Source: CAD feature listing. Evaluate the final solid. Frame: model axes, mm. A direction names the side the tool comes from. Coordinates: 2 decimals unless noted, no trailing zeros. Loops run counter-clockwise (first coordinate to the right, second up) from the corner with the lowest first, then second, coordinate; pieces in that order, holes last. Notation, with made-up numbers: M 7,-22.5 L 59,-22.5 A34 ccw 59,14.5 Z; hole C -15,16 d3. An arc over 180 degrees is marked long. One line per question, with ' | ' between items. Start each with the question number.
1. Section query C-C, the plane z = -0.5. Output: boundary loops of the cut face in (x, y).
2. Section query D-D, the plane x = -33. Output: boundary loops of the cut face in (y, z), and give its area (3 significant figures).
3. Mould query, pull axis Y, two halves, no side actions, for faces 4 (the flat face through (1, 80, -25)), 5 (the flat face through (-55, 32, -14)), 6 (the flat face through (26, 58, -16.876)), 7 (the cylindrical face through (20.24, 51.35, -14.34)). Classes: pulls with the +Y half, pulls with the -Y half, needs draft (parallel to the pull), parting line crosses it, or undercut.
4. Pin query (flat end, axial travel): P1, Ø5, axis at x = -19.5, y = 22, coming from the +Z side; P2, Ø15, axis at x = -1.5, y = 20, coming from the +Z side; P3, Ø8, axis at x = 0, y = 43, coming from the +Z side. Return the tip coordinate at first contact, or that it passes through.
5. Ray query, probe 1 along X at (y, z) = (25, 19.5); probe 2 along Y at (x, z) = (25, -30.5); probe 3 along Y at (x, z) = (25, -13.65). Return the intervals inside material, ascending.
6. Section query B-B, the plane x = 25. Output: boundary loops of the cut face in (y, z), and give its area (3 significant figures).
7. Section query A-A, the plane y = 55. Output: boundary loops of the cut face in (x, z), and give its area (3 significant figures).
8. Access query for faces 1 (the flat face through (-24, 58, -16.876)), 2 (the flat face through (20, 15, 9)), 3 (the flat face through (53.521, 15.21, 21.603)). Directions: +Z, -Z, +X, -X, +Y, -Y. A direction counts if a zero-diameter tool reaches every point of the face in a straight line with its end or side. Return the directions, or none.
```python
from build123d import *

# Parameters (mm, degrees)
BOSS_EXTRUDE2_DEPTH = 55
SKETCH4_W           = 40
SKETCH4_H           = 25
CUT_EXTRUDE1_DEPTH  = 83.974750358
SKETCH5_R           = 3
CUT_EXTRUDE2_DEPTH  = 104.198837203
SKETCH6_R           = 6
CUT_EXTRUDE3_DEPTH  = 5
CHAMFER1_SIZE       = 3


with BuildPart() as part:
    # Sketch3 → Boss-Extrude2 (new, symmetric)
    with BuildSketch(Plane(origin=(0, 0, 0), x_dir=(0, 0, -1), z_dir=(1, 0, 0))):
        Polygon((-23.124409198, 0), (36.875590802, 0), (36.875590802, 80), (11.875590802, 80), (11.875590802, 30), (-23.124409198, 30), align=None)
    extrude(amount=BOSS_EXTRUDE2_DEPTH, both=True)

    # Sketch4 → Cut-Extrude1 (cut, through all)
    with BuildSketch(Plane(origin=(0, 30, 0), x_dir=(1, 0, 0), z_dir=(0, 1, 0))):
        with Locations((0, -10.624409198)):
            Rectangle(SKETCH4_W, SKETCH4_H)
    extrude(amount=-CUT_EXTRUDE1_DEPTH, mode=Mode.SUBTRACT)

    # Sketch5 → Cut-Extrude2 (cut, through all)
    with BuildSketch(Plane.XY.offset(-11.875590802)):
        with Locations((-25, 55)):
            Circle(SKETCH5_R)
        with Locations((25, 55)):
            Circle(SKETCH5_R)
    extrude(amount=-CUT_EXTRUDE2_DEPTH, mode=Mode.SUBTRACT)

    # Sketch6 → Cut-Extrude3 (cut)
    with BuildSketch(Plane.XY.offset(-11.875590802)):
        with Locations((-25, 55)):
            Circle(SKETCH6_R)
        with Locations((25, 55)):
            Circle(SKETCH6_R)
    extrude(amount=-CUT_EXTRUDE3_DEPTH, mode=Mode.SUBTRACT)

    # Chamfer1
    chamfer1_edges = [part.edges().sort_by_distance(p)[0] for p in [
        (-20, 15, 23.124409198),
        (20, 15, 23.124409198),
        (55, 15, 23.124409198),
        (-55, 15, 23.124409198),
    ]]
    chamfer(chamfer1_edges, length=CHAMFER1_SIZE)


solid = part.part
```
Taken from the geometry:
1) outline: M -55,0 L -20,0 L -20,30 L -55,30 Z; M 20,0 L 55,0 L 55,30 L 20,30 Z
2) outline: M 0,-36.88 L 80,-36.88 L 80,-11.88 L 30,-11.88 L 30,23.12 L 0,23.12 Z | area: 3,050 mm^2
3) face 4: pulls with the +Y half | face 5: needs draft | face 6: undercut | face 7: undercut
4) P1: z = 22.12 | P2: z = -1.88 | P3: z = -11.88
5) probe 1: -55 to -20, 20 to 55 | probe 2: 0 to 52, 58 to 80 | probe 3: 0 to 49, 61 to 80
6) outline: M 0,-36.88 L 52,-36.88 L 52,-16.88 L 49,-16.88 L 49,-11.88 L 30,-11.88 L 30,23.12 L 0,23.12 Z; M 58,-36.88 L 80,-36.88 L 80,-11.88 L 61,-11.88 L 61,-16.88 L 58,-16.88 Z | area: 2,870 mm^2
7) outline: M -55,-36.88 L -28,-36.88 L -28,-16.88 L -31,-16.88 L -31,-11.88 L -55,-11.88 Z; M -22,-36.88 L 22,-36.88 L 22,-16.88 L 19,-16.88 L 19,-11.88 L -19,-11.88 L -19,-16.88 L -22,-16.88 Z; M 28,-36.88 L 55,-36.88 L 55,-11.88 L 31,-11.88 L 31,-16.88 L 28,-16.88 Z | area: 2,390 mm^2
8) face 1: +Z | face 2: +Z, +Y, -Y | face 3: +Z, +X, +Y, -Y
